from build123d import *

# Parameters (mm, degrees)
F1_DEPTH = 38.1
F3_DEPTH = 18.796
F5_DEPTH = 19.05
F6_R     = 9.8425
F7_DEPTH = 35.56


with BuildPart() as f1:
    # F0 (on Top) → F1 (new body)
    with BuildSketch(Plane.XY):
        Polygon((-12.0983748909, -20.955), (12.0983748909, -20.955), (24.1967497817, 0), (12.0983748909, 20.955), (-12.0983748909, 20.955), (-24.1967497817, 0), align=None)
    extrude(amount=F1_DEPTH)

    # F2 (on face) → F3 (join)
    with BuildSketch(Plane(origin=(0, 0, 0), x_dir=(1, 0, 0), z_dir=(0, 0, -1))):
        Polygon((-2.286, 20.955), (0, 20.955), (0, 23.241), (-3.429, 23.241), align=None)
        Polygon((0, 23.241), (0, 20.955), (2.286, 20.955), (3.429, 23.241), align=None)
    extrude(amount=-F3_DEPTH)

    # F4 (on face) → F5 (cut)
    with BuildSketch(Plane(origin=(0, 0, 0), x_dir=(1, 0, 0), z_dir=(0, 0, -1))):
        Polygon((15.9478578107, 9.2075), (18.1475623363, 10.4775), (16.8775623363, 12.6772045256), (14.0428578107, 12.5070567884), align=None)
        Polygon((19.4175623363, 8.2777954744), (18.1475623363, 10.4775), (15.9478578107, 9.2075), (17.8528578107, 5.9079432116), align=None)
    extrude(amount=-F5_DEPTH, mode=Mode.SUBTRACT)

    # F6 (on face) → F7 (cut)
    with BuildSketch(Plane.XY.offset(38.1)):
        with Locations((-6.0858491875, -10.541)):
            Circle(F6_R)
        with Locations((-6.0858491875, 10.541)):
            Circle(F6_R)
        with Locations((11.4346282032, 0)):
            Circle(F6_R)
    extrude(amount=-F7_DEPTH, mode=Mode.SUBTRACT)


solid = f1.part
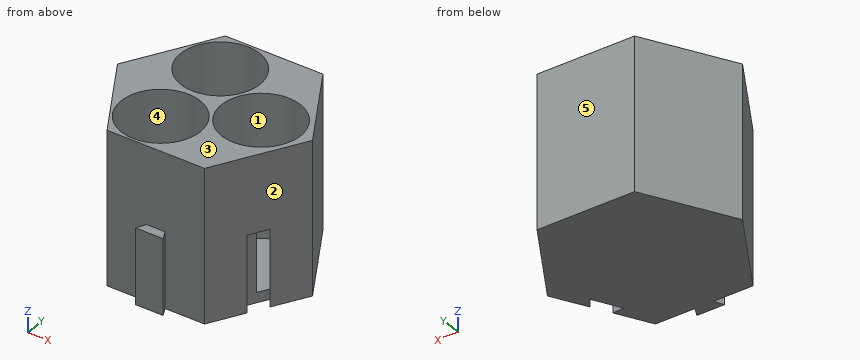
For this review, take the finished solid that the model builds, in its own axes (mm). Face numbers are marked on the shaded views. A direction names the side the tool comes from. Coordinates: 2 decimals unless noted, no trailing zeros. Order: outer loops, then holes, each group sorted by start corner. A loop starts at its lowest first (then second) coordinate and runs counter-clockwise, first axis right, second up. Notation, with made-up numbers: (78.5, 36.25) - (87.5, 36.25) arc R23 ccw to (87.5, 69.25) - close; hole circle Ø4 at (30.25, 66). An arc over 180 degrees is marked (long way). Answer as CSV lines item,"result". Start each with the question number.
1) Draft analysis for pull direction Y (two halves, no side actions). For the marked faces 1, 2 and 3, state which applies: +Y half, -Y half, draft (parallel to the pull), parting line (faces both ways), or undercut.
2) Machinability: for the marked faces 4 and 5, which of the approach directions +Z, -Z, +X, -X, +Y, -Y give a long, thin tool a straight path to every point of the face, cutting with its end or side? Answer none if there is none.
3) Add section C-C (z = 16). State the section outline as (x, y) points (1 decimal), then the cut area to 3 significant figures.
4) To check wall thickness, follow line 1 along Y through (x, z) = (-11.5, 9.5) (3 decimals); line 2 along X through (y, z) = (-9, 10); line 3 along X through (y, z) = (0, 13). State the ranges of each line that lie inside material, in increasing order. Write a range as [from, to].
5) Insertion check: P1, Ø1, axis at x = 1.5, z = 25, coming from the -Y side (3 decimals); P2, Ø5, axis at y = 14, z = 25.5, coming from the +X side; P3, Ø3, axis at y = -17, z = 5, coming from the +X side. Each pin has a flat end and moves straight along its axis. Give the tip position at first contact, or say it passes through.
6) Add section B-B (y = 12). State the section outline as (x, z) points.
7) Add section A-A (x = 15.5). State the section outline as (y, z) points, then the cut area to 3 significant figures.
8) Add section D-D (x = 10). State the section outline as (y, z) points (3 decimals), then the cut area to 3 significant figures.
Result:
1,face 1,"undercut"
1,face 2,"-Y half"
1,face 3,"draft"
2,face 4,"+Z"
2,face 5,"+Z, -Z, +X, -X, +Y"
3,outline,"(-24.2, 0) - (-12.1, -21) - (-2.3, -21) - (-3.4, -23.2) - (3.4, -23.2) - (2.3, -21) - (12.1, -21) - (16.9, -12.7) - (14, -12.5) - (16.3, -8.5) arc R9.8 cw (long way) to (18.5, -6.9) - (19.4, -8.3) - (24.2, 0) - (12.1, 21) - (-12.1, 21) - close; hole circle Ø19.7 at (-6.1, -10.5); hole circle Ø19.7 at (-6.1, 10.5)"
3,area,"607 mm^2"
4,line 1,"[-20.955, -18.761], [-2.321, 2.321], [18.761, 20.955]"
4,line 2,"[-19, -15.81], [3.64, 7.45], [15.42, 16.07]"
4,line 3,"[-24.2, 1.59], [21.28, 24.2]"
5,P1,"y = -20.955"
5,P2,"x = 17.56"
5,P3,"x = 15.25"
6,outline,"(-17.27, 0) - (17.27, 0) - (17.27, 38.1) - (3.65, 38.1) - (3.65, 2.54) - (-15.82, 2.54) - (-15.82, 38.1) - (-17.27, 38.1) - close"
7,outline,"(-15.06, 0) - (-12.59, 0) - (-12.59, 19.05) - (-9.98, 19.05) - (-9.98, 0) - (15.06, 0) - (15.06, 38.1) - (8.96, 38.1) - (8.96, 2.54) - (-8.96, 2.54) - (-8.96, 38.1) - (-15.06, 38.1) - close"
7,area,"461 mm^2"
8,outline,"(-20.955, 0) - (20.955, 0) - (20.955, 38.1) - (9.737, 38.1) - (9.737, 2.54) - (-9.737, 2.54) - (-9.737, 38.1) - (-20.955, 38.1) - close"
8,area,"904 mm^2"
